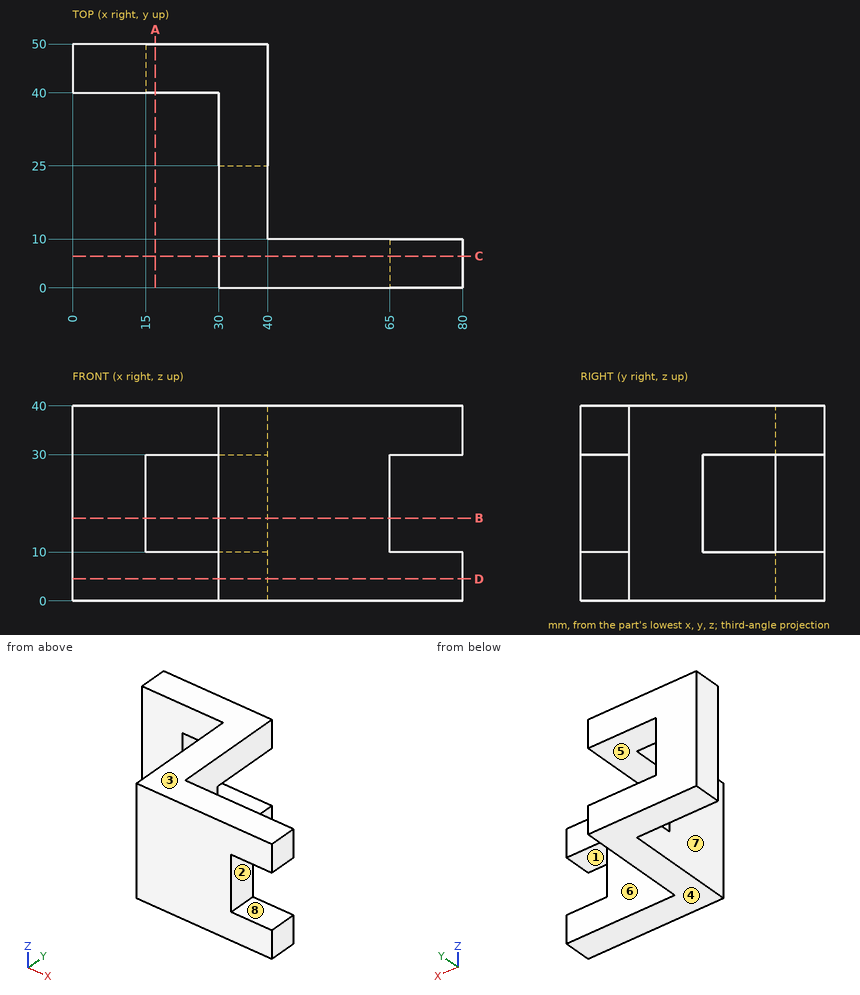
Verification items for this drawing (mm, ordinates from the low corner). A direction names the side the tool comes from. Coordinates: 2 decimals unless noted, no trailing zeros. Write each loop counter-clockwise with the first axis right and the second up, starting at its lowest first coordinate (ties: lowest second). Pieces come first, ordered by that corner, then holes. Notation, with made-up numbers: M 4.5,86 L 59.5,86 A21 cw 59.5,117 Z; hole C 39,29.25 d8. An arc over 180 degrees is marked long. Use CSV: the item, a comma, the result in double quotes.
Q1. Thickness scan on line 1 along Z through (x, y) = (29.5, 46); line 2 along X through (y, z) = (18, 20); line 3 along Y through (x, z) = (10, 24). Record the ranges inside material, lowest first. Write a range as [from, to].
Computed values:
line 1,"[0, 10], [30, 40]"
line 2,"[30, 40]"
line 3,"[40, 50]"
Q2. Section check A-A, the plane x = 17. Enter the section's corners in (y, z).
Computed values:
outline,"M 40,0 L 50,0 L 50,10 L 40,10 Z; M 40,30 L 50,30 L 50,40 L 40,40 Z"
Q3. Set-up check for the marked faces 5, 6, 7 and 8: record each of +Z, -Z, +X, -X, +Y, -Y from which the full face is reachable in a straight line by a thin tool's end or side.
Computed values:
face 5,"+X, +Y"
face 6,"+Z, -Z, +X, +Y"
face 7,"+Z, -Z, -X, -Y"
face 8,"+X, +Y, -Y"
Q4. Section check B-B, the plane z = 17. Enter the section's corners in (x, y).
Computed values:
outline,"M 0,40 L 15,40 L 15,50 L 0,50 Z; M 30,0 L 65,0 L 65,10 L 40,10 L 40,25 L 30,25 Z"
Q5. Mould release check, pull along Z, two halves, no side actions. Record for the marked faces 1, 2, 3 and 4: pulls with the +Z half, pulls with the -Z half, needs draft (parallel to the pull), parting line crosses it, or undercut.
Computed values:
face 1,"undercut"
face 2,"undercut"
face 3,"pulls with the +Z half"
face 4,"pulls with the -Z half"
Q6. Go/stop test with flat-tipped pins: P1, Ø5, axis at y = 24.5, z = 32.5, coming from the +X side; P2, Ø4, axis at y = 5.5, z = 13, coming from the -X side; P3, Ø1.5, axis at x = 36, z = 17.5, coming from the +Y side. Record where each tip stops, or that it passes through.
Computed values:
P1,"x = 40"
P2,"x = 30"
P3,"y = 25"
Q7. Section check C-C, the plane y = 6.5. Enter the section's corners in (x, z).
Computed values:
outline,"M 30,0 L 80,0 L 80,10 L 65,10 L 65,30 L 80,30 L 80,40 L 30,40 Z"
Q8. Section check D-D, the plane z = 4.5. Enter the section's corners in (x, y), and give its area (3 significant figures).
Computed values:
outline,"M 0,40 L 30,40 L 30,0 L 80,0 L 80,10 L 40,10 L 40,50 L 0,50 Z"
area,"1,200 mm²"
